Verification items for the finished model (mm, model axes). A direction names the side the tool comes from. Coordinates: 2 decimals unless noted, no trailing zeros. Write each loop counter-clockwise with the first axis right and the second up, starting at its lowest first coordinate (ties: lowest second). Pieces come first, ordered by that corner, then holes. Notation, with made-up numbers: M 43,52 L 101,52 A15 ccw 101,74 Z; hole C -15,-30.5 d5. An arc over 180 degrees is marked long. Answer in a Markdown table with one row per item.
from build123d import *

# Parameters (mm, degrees)
F0_W         = 131.8914890289
F0_H         = 55.0068765879
F1_DEPTH     = 44.958
F2_T         = -2.54
F3_W         = 33.3715188317
F3_H         = 6.021162495
F4_DEPTH     = 10.922
F5_W         = 6.7100599408
F5_H         = 29.552442953
F6_DEPTH     = 25.4
F7_T1_DEPTH  = 48.7017749528
F8_W         = 30.4629029706
F8_H         = 4.9823708832
F9_DEPTH     = 8.128
F10_W        = 5.0006210804
F10_H        = 27.0441961475
F11_DEPTH    = 25.4
F12_T1_DEPTH = 45.7931590917


# Not quite as in the source:
# - a fillet or chamfer that OpenCascade refuses, or shapes differently, is made with other operations: its cross-section is extruded or revolved along the edge and cut away or added


with BuildPart() as f1:
    # F0 (on Top) → F1 (new body)
    with BuildSketch(Plane.XY):
        with Locations((0.1562684774, 11.095136404)):
            Rectangle(F0_W, F0_H)
    extrude(amount=F1_DEPTH)

    # F2
    f2_openings = [f1.faces().sort_by_distance(p)[0] for p in [
        (0.156268, 11.095136, 44.958),
    ]]
    offset(amount=F2_T, openings=f2_openings)

    # F3 (on face) → F4 (join)
    with BuildSketch(Plane.YZ.offset(66.1020129919)):
        with Locations((12.0295642409, 32.4530350044)):
            Rectangle(F3_W, F3_H)
    extrude(amount=F4_DEPTH)

    # F5 (on face) → F6 (cut)
    with BuildSketch(Plane.XY.offset(35.4636162519)):
        with Locations((71.2361820042, 11.8320556358)):
            Rectangle(F5_W, F5_H)
    extrude(amount=-F6_DEPTH, mode=Mode.SUBTRACT)

    # F7: fillet of radius 3.0660512242 on 2 edges, made by hand

    # F7_s2 → F7_t1 (cut)
    with BuildSketch(Plane.XZ.offset(-36.3804517173)):
        with BuildLine():
            ThreePointArc((73.9579617677, 35.4636162519), (76.1259873798, 34.5655906398), (77.0240129919, 32.3975650277))
            Line((77.0240129919, 32.3975650277), (77.0240129919, 35.4636162519))
            Line((77.0240129919, 35.4636162519), (73.9579617677, 35.4636162519))
        make_face()
        with BuildLine():
            ThreePointArc((73.9579617677, 29.4424537569), (76.1259873798, 30.340479369), (77.0240129919, 32.5085049811))
            Line((77.0240129919, 32.5085049811), (77.0240129919, 29.4424537569))
            Line((77.0240129919, 29.4424537569), (73.9579617677, 29.4424537569))
        make_face()
    extrude(amount=F7_T1_DEPTH, mode=Mode.SUBTRACT)

    # F8 (on face) → F9 (join)
    with BuildSketch(Plane(origin=(-65.789476037, 0, 0), x_dir=(0, -1, 0), z_dir=(-1, 0, 0))):
        with Locations((-11.8714510463, 30.9710260481)):
            Rectangle(F8_W, F8_H)
    extrude(amount=F9_DEPTH)

    # F10 (on face) → F11 (cut)
    with BuildSketch(Plane.XY.offset(33.4622114897)):
        with Locations((-69.5076957345, 11.8382142391)):
            Rectangle(F10_W, F10_H)
    extrude(amount=-F11_DEPTH, mode=Mode.SUBTRACT)

    # F12: fillet of radius 3.0660512242 on 2 edges, made by hand

    # F12_s2 → F12_t1 (cut)
    with BuildSketch(Plane.XZ.offset(-34.7680305922)):
        with BuildLine():
            ThreePointArc((-70.8514248128, 33.4622114897), (-73.0194504249, 32.5641858776), (-73.917476037, 30.3961602655))
            Line((-73.917476037, 30.3961602655), (-73.917476037, 33.4622114897))
            Line((-73.917476037, 33.4622114897), (-70.8514248128, 33.4622114897))
        make_face()
        with BuildLine():
            ThreePointArc((-70.8514248128, 28.4798406065), (-73.0194504249, 29.3778662186), (-73.917476037, 31.5458918307))
            Line((-73.917476037, 31.5458918307), (-73.917476037, 28.4798406065))
            Line((-73.917476037, 28.4798406065), (-70.8514248128, 28.4798406065))
        make_face()
    extrude(amount=F12_T1_DEPTH, mode=Mode.SUBTRACT)


solid = f1.part
1) Sectioned sample at A-A (y = 6). Record the cut outline in (x, z), then the cut area to 3 significant figures.
Response values:
| item | result |
|---|---|
| outline | M -73.86,30.97 A3.07 ccw -72.01,28.71 L -72.01,33.24 A3.07 ccw Z; M -67.01,28.48 L -65.79,28.48 L -65.79,0 L 66.1,0 L 66.1,29.44 L 67.88,29.44 L 67.88,35.46 L 66.1,35.46 L 66.1,44.96 L 63.56,44.96 L 63.56,2.54 L -63.25,2.54 L -63.25,44.96 L -65.79,44.96 L -65.79,33.46 L -67.01,33.46 Z; M 74.59,29.51 A3.07 ccw 77.02,32.45 A3.07 ccw 74.59,35.4 Z |
| area | 584 mm² |
2) Sectioned sample at C-C (z = 20). Record the cut outline in (x, y), then the cut area to 3 significant figures.
Response values:
| item | result |
|---|---|
| outline | M -65.79,-16.41 L 66.1,-16.41 L 66.1,38.6 L -65.79,38.6 Z; hole M -63.25,-13.87 L 63.56,-13.87 L 63.56,36.06 L -63.25,36.06 Z |
| area | 924 mm² |
3) Tool access check on faces 1 (the face through (-70, -3.36, 31)), 2 (the face through (-70, 27.103, 31)), 3 (the face through (-72.008, 12, 31)), 4 (the face through (-1, 11, 2.54)). Record the directions out of +Z, -Z, +X, -X, +Y, -Y that give a thin tool (end or side, any length) a straight path to the whole face; none if there is none.
Response values:
| item | result |
|---|---|
| face 1 | +Z, -Z, -X, -Y |
| face 2 | +Z, -Z, -X, +Y |
| face 3 | +Z, -Z |
| face 4 | +Z |
4) Release check for a two-part mould opening along Y. For faces 5 (the face through (71, 28.715, 32)), 6 (the face through (-1, -16.408, 22)), 7 (the face through (71, -2.944, 32)), 8 (the face through (67, 12, 29.442)) record: +Y half, -Y half, draft (parallel to the pull), parting line (faces both ways), or undercut.
Response values:
| item | result |
|---|---|
| face 5 | +Y half |
| face 6 | -Y half |
| face 7 | undercut |
| face 8 | draft |
5) Sectioned sample at D-D (y = -11). Record the cut outline in (x, z), then the cut area to 3 significant figures.
Response values:
| item | result |
|---|---|
| outline | M -65.79,0 L 66.1,0 L 66.1,44.96 L 63.56,44.96 L 63.56,2.54 L -63.25,2.54 L -63.25,44.96 L -65.79,44.96 Z |
| area | 550 mm² |
6) Depth check by flat-ended pin: pin 1 (1.5 mm diameter, centred on y = -4, z = 6, fed in from -X); pin 2 (10 mm diameter, centred on x = 54.5, y = 3, fed in from +Z); pin 3 (2 mm diameter, centred on y = -7, z = 5.5, fed in from +X). Enter the tip coordinate at first touch or a pass-through.
Response values:
| item | result |
|---|---|
| pin 1 | stops at x = -65.79 |
| pin 2 | stops at z = 2.54 |
| pin 3 | stops at x = 66.1 |
7) Thickness scan on L1, parallel to X at y = 25.5, z = 13.5; L2, parallel to Y at x = -20.5, z = 15.5; L3, parallel to X at y = 13.5, z = 29. Record the ranges inside material, lowest first. Write a range as [from, to].
Response values:
| item | result |
|---|---|
| L1 | x = [-65.79, -63.25], [63.56, 66.1] |
| L2 | y = [-16.41, -13.87], [36.06, 38.6] |
| L3 | x = [-72.56, -72.01], [-67.01, -63.25], [63.56, 66.1] |
8) Sectioned sample at B-B (x = -39.5). Record the cut outline in (y, z), then the cut area to 3 significant figures.
Response values:
| item | result |
|---|---|
| outline | M -16.41,0 L 38.6,0 L 38.6,44.96 L 36.06,44.96 L 36.06,2.54 L -13.87,2.54 L -13.87,44.96 L -16.41,44.96 Z |
| area | 355 mm² |
